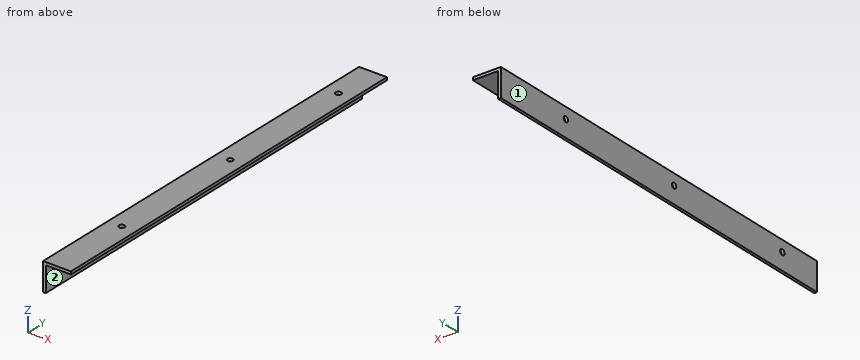
from build123d import *

# Parameters (mm, degrees)
BOSS_EXTRUDE1_DEPTH      = 146
BOSS_EXTRUDE1_DEPTH_BACK = 146
SKETCH2_R                = 2
CUT_EXTRUDE1_DEPTH       = 10
SKETCH3_R                = 2
CUT_EXTRUDE2_DEPTH       = 10


with BuildPart() as part:
    # Sketch1 → Boss-Extrude1 (new, two sides: drawn at the far end of the back side and taken through both)
    with BuildSketch(Plane(origin=(0, 0, 0), x_dir=(1, 0, 0), z_dir=(0, 1, 0)).offset(-BOSS_EXTRUDE1_DEPTH_BACK)):
        Polygon((0, 0), (20, 0), (20, 2), (2, 2), (2, 20), (0, 20), align=None)
    extrude(amount=BOSS_EXTRUDE1_DEPTH + BOSS_EXTRUDE1_DEPTH_BACK)

    # Sketch2 → Cut-Extrude1 (cut)
    with BuildSketch(Plane.XY):
        with Locations((10, 114)):
            Circle(SKETCH2_R)
        with Locations((10, 14)):
            Circle(SKETCH2_R)
        with Locations((10, -86)):
            Circle(SKETCH2_R)
    extrude(amount=-CUT_EXTRUDE1_DEPTH, mode=Mode.SUBTRACT)

    # Sketch3 → Cut-Extrude2 (cut)
    with BuildSketch(Plane.ZY):
        with Locations((-8, -114)):
            Circle(SKETCH3_R)
        with Locations((-8, -14)):
            Circle(SKETCH3_R)
        with Locations((-8, 86)):
            Circle(SKETCH3_R)
    extrude(amount=-CUT_EXTRUDE2_DEPTH, mode=Mode.SUBTRACT)


solid = part.part
For this review, take the finished solid that the model builds, in its own axes (mm). Face numbers are marked on the shaded views. A direction names the side the tool comes from. Give positions to 0.01 mm unless a question says otherwise; leave off trailing zeros. Loops run counter-clockwise (first coordinate to the right, second up) from the corner with the lowest first, then second, coordinate; pieces in that order, holes last. Notation, with made-up numbers: (69, -5) -> (121, -5) arc R7 ccw to (121, 0) -> close; hole circle Ø7 at (-35, 20). An arc over 180 degrees is marked (long way). One line per question, with ' | ' between items.
1) We need section B-B (z = -17). Write out the cut boundary in (x, y).
Resolved:
outline: (0, -146) -> (2, -146) -> (2, 146) -> (0, 146) -> close
2) For the marked faces 1 and 2, list the 3-axis set-ups (+Z, -Z, +X, -X, +Y, -Y) from which the entire face can be reached by the end or side of a thin tool; tool diameter is ignored.
Resolved:
face 1: +Z, -Z, -X, +Y, -Y | face 2: -Z, +X, +Y, -Y
3) We need section A-A (y = -101.5). Write out the cut boundary in (x, z), plus the area to 3 significant figures.
Resolved:
outline: (0, -20) -> (2, -20) -> (2, -2) -> (20, -2) -> (20, 0) -> (0, 0) -> close | area: 76.0 mm2
4) To check wall thickness, follow probe 1 along Y at (x, z) = (10, -0.7); probe 2 along Y at (x, z) = (0.7, -8); probe 3 along X at (y, z) = (108.5, -7.25). State the ranges of each line that lie inside material, in increasing order.
Resolved:
probe 1: y = -146 to -88, -84 to 12, 16 to 112, 116 to 146 | probe 2: y = -146 to -116, -112 to -16, -12 to 84, 88 to 146 | probe 3: x = 0 to 2
5) Insertion check: pin 1 Ø3.5 at (y, z) = (-114, -8) entering from +X; pin 2 Ø6.5 at (y, z) = (-14, -8) entering from +X; pin 3 Ø5.5 at (x, y) = (11, 47) entering from -Z. Each pin has a flat end and moves straight along its axis. Give the tip position at first contact, or say it passes through.
Resolved:
pin 1: passes through | pin 2: stops at x = 2 | pin 3: stops at z = -2
